from build123d import *

# Parameters (mm, degrees)
SKETCH1_R           = 27.001022249
BOSS_EXTRUDE1_DEPTH = 10
SKETCH2_R           = 17.811284506
BOSS_EXTRUDE3_DEPTH = 4
SKETCH3_R           = 11.844355023
CUT_EXTRUDE2_DEPTH  = 41.67075614
FILLET1_R           = 2


with BuildPart() as part:
    # Sketch1 → Boss-Extrude1 (new body)
    with BuildSketch(Plane(origin=(0, 0, 0), x_dir=(1, 0, 0), z_dir=(0, 1, 0))):
        with Locations(Location((0, 0, 0), (0, 0, 270))):
            Circle(SKETCH1_R)
    extrude(amount=BOSS_EXTRUDE1_DEPTH)

    # Sketch2 → Boss-Extrude3 (add)
    with BuildSketch(Plane(origin=(0, 10, 0), x_dir=(1, 0, 0), z_dir=(0, 1, 0))):
        with Locations(Location((0, 0, 0), (0, 0, 270))):
            Circle(SKETCH2_R)
    extrude(amount=BOSS_EXTRUDE3_DEPTH)

    # Sketch3 → Cut-Extrude2 (cut, through all)
    with BuildSketch(Plane(origin=(0, 14, 0), x_dir=(1, 0, 0), z_dir=(0, 1, 0))):
        with Locations(Location((0, 0, 0), (0, 0, 270))):
            Circle(SKETCH3_R)
    extrude(amount=-CUT_EXTRUDE2_DEPTH, mode=Mode.SUBTRACT)

    # Fillet1
    fillet1_edges = [part.edges().sort_by_distance(p)[0] for p in [
        (0, 10, -27.001022249),
        (0, 10, -17.811284506),
    ]]
    fillet(fillet1_edges, radius=FILLET1_R)


solid = part.part
Verification items for the finished model (mm, model axes). A direction names the side the tool comes from. Coordinates: 2 decimals unless noted, no trailing zeros. Loops run counter-clockwise (first coordinate to the right, second up) from the corner with the lowest first, then second, coordinate; pieces in that order, holes last. Notation, with made-up numbers: (56, 24.25) -> (80, 24.25) arc R12 cw to (80, 44.25) -> close; hole circle Ø2 at (89, -4.5). An arc over 180 degrees is marked (long way). Write each question's results on one line, items separated by ' | '.
Item 1: Gauge pin test, flat ends, axial feed: pin 1 (8 mm diameter, centred on y = 4.5, z = 9, fed in from +X); pin 2 (8 mm diameter, centred on x = 4.5, y = 5, fed in from +Z); pin 3 (8 mm diameter, centred on y = 12, z = -17.5, fed in from +X). Record the tip position at first contact, or that the pin passes through.
Found:
pin 1: stops at x = 26.53 | pin 2: stops at z = 27 | pin 3: stops at x = 22.23
Item 2: Mould release check, pull along X, two halves, no side actions. Record for faces 1 (the face through (-12, 14, 4)), 2 (the face through (-11.563, 7.098, -2.568)), 3 (the face through (5.35, 12.99, 16.99)): +X half, -X half, draft (parallel to the pull), parting line (faces both ways), or undercut.
Found:
face 1: draft | face 2: undercut | face 3: parting line
Item 3: Section check B-B, the plane y = 12.75. Enter the section's corners in (x, z), plus the area to 3 significant figures.
Found:
outline: circle Ø35.62 at (0, 0); hole circle Ø23.69 at (0, 0) | area: 556 mm2
Item 4: Tool access check on faces 4 (the face through (19, 10, -8)), 5 (the face through (-6, 0, 12)). Record the directions out of +Z, -Z, +X, -X, +Y, -Y that give a thin tool (end or side, any length) a straight path to the whole face; none if there is none.
Found:
face 4: +Y | face 5: +Z, -Z, +X, -X, -Y
Item 5: Section check C-C, the plane y = 2.25. Enter the section's corners in (x, z), plus the area to 3 significant figures.
Found:
outline: circle Ø54 at (0, 0); hole circle Ø23.69 at (0, 0) | area: 1,850 mm2
Item 6: Section check A-A, the plane z = 0. Enter the section's corners in (x, y), plus the area to 3 significant figures.
Found:
outline: (-27, 0) -> (-11.84, 0) -> (-11.84, 14) -> (-17.81, 14) -> (-17.81, 12) arc R2 cw to (-19.81, 10) -> (-25, 10) arc R2 ccw to (-27, 8) -> close; (11.84, 0) -> (27, 0) -> (27, 8) arc R2 ccw to (25, 10) -> (19.81, 10) arc R2 cw to (17.81, 12) -> (17.81, 14) -> (11.84, 14) -> close | area: 351 mm2
Item 7: Material ranges on L1, parallel to X at y = 5.25, z = 0; L2, parallel to X at y = 8.75, z = 8.5; L3, parallel to Z at x = -10.5, y = 6, recorded low to high.
Found:
L1: x = -27 to -11.84, 11.84 to 27 | L2: x = -25.47 to -8.25, 8.25 to 25.47 | L3: z = -24.88 to -5.48, 5.48 to 24.88
